Geometry check sheet. Reference: the model listing, model coordinates, mm. A direction names the side the tool comes from. Round coordinates to 2 decimals unless told otherwise and drop trailing zeros. Loops run counter-clockwise (first coordinate to the right, second up) from the corner with the lowest first, then second, coordinate; pieces in that order, holes last. Notation, with made-up numbers: (23, 43) - (56, 43) arc R35 cw to (56, 79) - close; hole circle Ø7 at (71.25, 79.5). An arc over 180 degrees is marked (long way). Answer as CSV lines item,"result". Start each with the question number.
1) Draft check along Y on faces 1 (the flat face through (0, 7, -1)), 2 (the flat face through (0, 11, 1)), 3 (the flat face through (15, -4.9, -0.5)), 4 (the cylindrical face through (-12.606, 1.588, 0.986)). Enter one of: released by +Y, released by -Y, zero draft, split by the parting line, or undercut.
2) Cross-section at C-C on x = -4. Record the boundary of the cut face in (y, z).
3) Depth check by flat-ended pin: P1, Ø5, axis at x = 10.5, y = -0.5, coming from the -Z side. Enter the tip coordinate at first touch or a pass-through.
4) Thickness scan on line 1 along Y through (x, z) = (-20, 1.4); line 2 along X through (y, z) = (0.75, 1.7); line 3 along Y through (x, z) = (2, 0.7). Record the ranges inside material, lowest first.
5) Cross-section at D-D on x = 10. Record the boundary of the cut face in (y, z).
6) Cross-section at B-B on y = -9.5. Record the boundary of the cut face in (x, z).
7) Cross-section at A-A on y = 1.5. Record the boundary of the cut face in (x, z).
8) Access from +Z, -Z, +X, -X, +Y, -Y to the whole of each face (thin tool, end or side, straight path). Record for faces 5 (the flat face through (23, -3, 1)), 6 (the flat face through (0, -12, 1)), 7 (the flat face through (0.2, 6, -0.5)).
from build123d import *

# Parameters (mm, degrees)
CROQUIS1_W          = 30
CROQUIS1_H          = 11
CROQUIS1_R          = 2
UNION_IMU_DEPTH     = 2
CROQUIS2_R          = 1.75
UNION_CARCASA_DEPTH = 3


with BuildPart() as part:
    # Croquis1 → union-imu (new body)
    with BuildSketch(Plane.XY):
        with Locations((0, 0.5)):
            Rectangle(CROQUIS1_W, CROQUIS1_H)
        with Locations((-10.607695155, 1.5)):
            Circle(CROQUIS1_R, mode=Mode.SUBTRACT)
        with Locations((10.392304845, 1.5)):
            Circle(CROQUIS1_R, mode=Mode.SUBTRACT)
    extrude(amount=UNION_IMU_DEPTH)

    # Croquis2 → union-carcasa (add)
    with BuildSketch(Plane.XY.offset(2)):
        Polygon((-23, -17), (23, -17), (23, -4), (23, 11), (-23, 11), (-23, -4), align=None)
        with Locations((20, -3)):
            Circle(CROQUIS2_R, mode=Mode.SUBTRACT)
        with Locations((-20, -3)):
            Circle(CROQUIS2_R, mode=Mode.SUBTRACT)
        Polygon((15, -12), (15, -5), (15, 6), (-15, 6), (-15, -5), (-15, -12), align=None, mode=Mode.SUBTRACT)
    extrude(amount=-UNION_CARCASA_DEPTH)


solid = part.part
Answer block:
1,face 1,"zero draft"
1,face 2,"released by +Y"
1,face 3,"undercut"
1,face 4,"undercut"
2,outline,"(-17, -1) - (-12, -1) - (-12, 2) - (-17, 2) - close; (-5, 0) - (6, 0) - (6, -1) - (11, -1) - (11, 2) - (-5, 2) - close"
3,P1,"stops at z = 0"
4,line 1,"y = -17 to -4.75, -1.25 to 11"
4,line 2,"x = -23 to -12.46, -8.75 to 8.54, 12.25 to 23"
4,line 3,"y = -17 to -12, -5 to 11"
5,outline,"(-17, -1) - (-12, -1) - (-12, 2) - (-17, 2) - close; (-5, 0) - (-0.46, 0) - (-0.46, 2) - (-5, 2) - close; (3.46, 0) - (6, 0) - (6, -1) - (11, -1) - (11, 2) - (3.46, 2) - close"
6,outline,"(-23, -1) - (-15, -1) - (-15, 2) - (-23, 2) - close; (15, -1) - (23, -1) - (23, 2) - (15, 2) - close"
7,outline,"(-23, -1) - (-15, -1) - (-15, 0) - (-12.61, 0) - (-12.61, 2) - (-23, 2) - close; (-8.61, 0) - (8.39, 0) - (8.39, 2) - (-8.61, 2) - close; (12.39, 0) - (15, 0) - (15, -1) - (23, -1) - (23, 2) - (12.39, 2) - close"
8,face 5,"+Z, -Z, +X, +Y, -Y"
8,face 6,"+Z, -Z"
8,face 7,"-Z"
